Study the drawing (mm; zero at the part's minimum x, y, z) and answer. Give positions to 0.01 mm unless a question says otherwise; leave off trailing zeros. Order: outer loops, then holes, each group sorted by start corner. A loop starts at its lowest first (then second) coordinate and runs counter-clockwise, first axis right, second up. Notation, with made-up numbers: (-7, -26.75) - (18, -26.75) arc R25 ccw to (18, -1.75) - close; hole circle Ø8 at (29.25, 79.25). An arc over 180 degrees is marked (long way). Put each result on its own line as item: value.
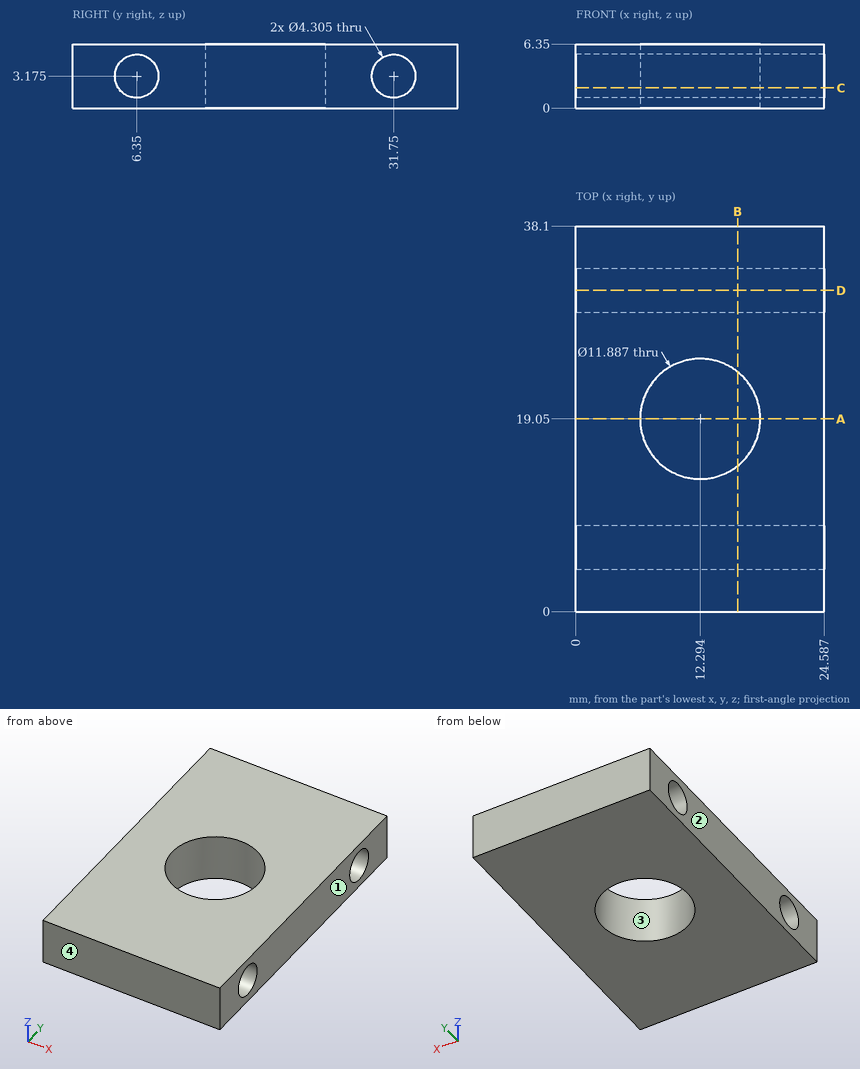
(1) Section C-C, the plane z = 2 is taken. Write down the section's boundary in (x, y).
Geometry check:
outline: (0, 0) - (24.59, 0) - (24.59, 4.55) - (0, 4.55) - close; (0, 8.15) - (24.59, 8.15) - (24.59, 29.95) - (0, 29.95) - close; (0, 33.55) - (24.59, 33.55) - (24.59, 38.1) - (0, 38.1) - close; hole circle Ø11.89 at (12.29, 19.05)
(2) Section D-D, the plane y = 31.75 is taken. Write down the section's boundary in (x, z).
Geometry check:
outline: (0, 0) - (24.59, 0) - (24.59, 1.02) - (0, 1.02) - close; (0, 5.33) - (24.59, 5.33) - (24.59, 6.35) - (0, 6.35) - close
(3) Section A-A, the plane y = 19.05 is taken. Write down the section's boundary in (x, z).
Geometry check:
outline: (0, 0) - (6.35, 0) - (6.35, 6.35) - (0, 6.35) - close; (18.24, 0) - (24.59, 0) - (24.59, 6.35) - (18.24, 6.35) - close
(4) Given pin 1 (7 mm diameter, centred on x = 12.29, y = 19.05, fed in from +Z), flat-ended and moving along its own axis, determine where the tip first touches the part or whether it passes through.
Geometry check:
pin 1: passes through
(5) Determine the mould class of the marked faces 1, 2, 3 and 4 for opening direction X: pulls with the +X half, pulls with the -X half, needs draft (parallel to the pull), parting line crosses it, or undercut.
Geometry check:
face 1: pulls with the +X half
face 2: pulls with the -X half
face 3: undercut
face 4: needs draft
(6) Section B-B, the plane x = 16 is taken. Count the separate pieces of the cut face and the enclosed holes in it, then the cut area to 3 significant figures.
Geometry check:
separate pieces: 2
enclosed holes: 2
area: 154 mm²
(7) Straight lines are drawn through the part: line 1 (Y direction, x = 5.5, z = 2.5) (1 decimal); line 2 (Y direction, x = 15, z = 2.5) (1 decimal); line 3 (Y direction, x = 20, z = 5) (1 decimal). For each, find the intervals that lie inside material, in ascending order.
Geometry check:
line 1: y = 0 to 4.3, 8.4 to 29.7, 33.8 to 38.1
line 2: y = 0 to 4.3, 8.4 to 13.8, 24.3 to 29.7, 33.8 to 38.1
line 3: y = 0 to 5.2, 7.5 to 30.6, 32.9 to 38.1
